Read the model definition and answer for the solid it produces. Units are mm, in the model's axes. Face numbers are marked on the shaded views. A direction names the side the tool comes from. Coordinates: 2 decimals unless noted, no trailing zeros. One line per question, with ' | ' between items. Start each with the question number.
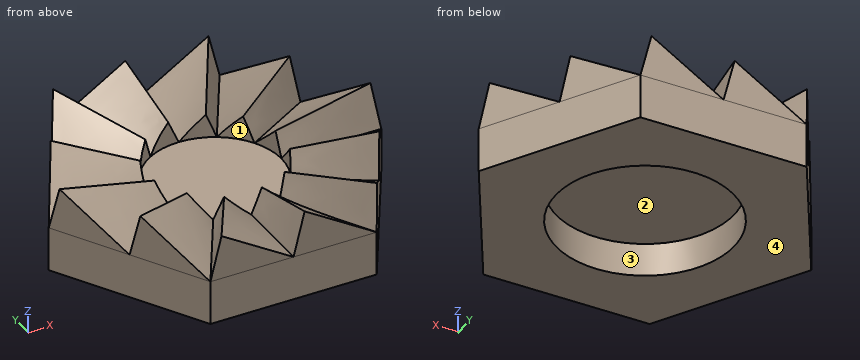
```python
from build123d import *

# Parameters (mm, degrees)
F1_DEPTH        = 2
F6_COPIES_COUNT = 6
F7_COPIES_COUNT = 6
F8_R            = 4
F9_DEPTH        = 1.5
F10_R           = 3
F11_DEPTH       = 2.0010001


# Not quite as in the source:
# - a pattern or mirror of a feature is missing from the dataset's text; its kind, count and spacing are read off the source's solid


with BuildPart() as f1:
    # F0 (on Top) → F1 (new body)
    with BuildSketch(Plane.XY):
        Polygon((3.7527767497, 6.5), (-3.7527767497, 6.5), (-7.5055534995, 0), (-3.7527767497, -6.5), (3.7527767497, -6.5), (7.5055534995, 0), align=None)
    extrude(amount=F1_DEPTH)

    # F5 (on offset) → F6 section 0
    with BuildSketch(Plane(origin=(-2.1650635095, -1.25, 0), x_dir=(0.5, -0.8660254038, 0), z_dir=(-0.8660254038, -0.5, 0))):
        Polygon((-0.943375673, 3), (-1.443375673, 2), (0, 2), align=None)
    # F3 (on face) → F6 section 1
    with BuildSketch(Plane(origin=(-5.6291651246, -3.25, 0), x_dir=(0.5, -0.8660254038, 0), z_dir=(-0.8660254038, -0.5, 0))):
        Polygon((-3.2527767497, 4), (-3.7527767497, 2), (0, 2), align=None)
    f6 = loft()

    # F6_copies: F6 ×6 about axis
    f6_copies_axis = Axis((0, 0, 0), (0, 0, 1))
    for i in range(1, F6_COPIES_COUNT):
        add(f6.rotate(f6_copies_axis, i * 360 / F6_COPIES_COUNT))

    # F5 (on offset) → F7 section 0
    with BuildSketch(Plane(origin=(-2.1650635095, -1.25, 0), x_dir=(0.5, -0.8660254038, 0), z_dir=(-0.8660254038, -0.5, 0))):
        Polygon((0.5, 3), (0, 2), (1.443375673, 2), align=None)
    # F3 (on face) → F7 section 1
    with BuildSketch(Plane(origin=(-5.6291651246, -3.25, 0), x_dir=(0.5, -0.8660254038, 0), z_dir=(-0.8660254038, -0.5, 0))):
        Polygon((0.5, 4), (0, 2), (3.7527767497, 2), align=None)
    f7 = loft()

    # F7_copies: F7 ×6 about axis
    f7_copies_axis = Axis((0, 0, 0), (0, 0, 1))
    for i in range(1, F7_COPIES_COUNT):
        add(f7.rotate(f7_copies_axis, i * 360 / F7_COPIES_COUNT))

    # F8 (on Top) → F9 (cut)
    with BuildSketch(Plane.XY):
        Circle(F8_R)
    extrude(amount=F9_DEPTH, mode=Mode.SUBTRACT)

    # F10 (on face) → F11 (cut, through all)
    with BuildSketch(Plane.XY.offset(2)):
        Circle(F10_R)
    extrude(amount=F11_DEPTH, mode=Mode.SUBTRACT)


solid = f1.part
```
(1) A tool of negligible diameter and unlimited length cuts with its end or side. For the marked faces 1 and 2, from which of +Z, -Z, +X, -X, +Y, -Y can it reach the whole face along a straight path? Write none if from no direction.
(2) Each of these flat-tipped pins is pushed along its axis until it touches: pin 1 Ø5 at (x, y) = (0, 0) entering from -Z; pin 2 Ø3 at (x, y) = (-0.5, 0) entering from +Z; pin 3 Ø2 at (y, z) = (1.5, 3) entering from -X. Where does it stop, or does it pass through?
(3) Section A-A on z = 3.5 is taken. Give the number of separate pieces and of enclosed holes in the cut face, plus the area to 3 significant figures.
(4) Find the intervals of material crossed by probe 1 along Y at (x, z) = (0, 0.8); probe 2 along Y at (x, z) = (-4, 3.15); probe 3 along Z at (x, y) = (1, -4), in increasing order. Write a range as from..to.
(5) Determine the mould class of the marked faces 3 and 4 for opening direction X: +X half, -X half, draft (parallel to the pull), parting line (faces both ways), or undercut.
Working result:
1) face 1: +Z | face 2: -Z
2) pin 1: stops at z = 1.5 | pin 2: stops at z = 2 | pin 3: stops at x = -7.13
3) separate pieces: 12 | enclosed holes: 0 | area: 11.0 mm2
4) probe 1: y = -6.5..-4, 4..6.5 | probe 2: y = -3.9..-2.73, -0.62..-0.39, 1.33..1.86, 4.36..6.07 | probe 3: z = 0..3
5) face 3: undercut | face 4: draft
